Geometry check sheet. Reference: the model listing, model coordinates, mm. Face numbers are marked on the shaded views. Coordinates: 2 decimals unless noted, no trailing zeros. Write each loop counter-clockwise with the first axis right and the second up, starting at its lowest first coordinate (ties: lowest second). Pieces come first, ordered by that corner, then holes.
from build123d import *

# Parameters (mm, degrees)
SKETCH1_R           = 14
SKETCH1_R_2         = 5
BOSS_EXTRUDE1_DEPTH = 38
SKETCH2_R           = 8
SKETCH2_R_2         = 3
BOSS_EXTRUDE2_DEPTH = 16
SKETCH3_R           = 2.5
CUT_EXTRUDE1_DEPTH  = 21
SKETCH4_R           = 2.15
SKETCH4_R_2         = 2.5
CUT_EXTRUDE2_DEPTH  = 21
CUT_EXTRUDE3_DEPTH  = 1
FILLET2_R           = 0.2


with BuildPart() as part:
    # Sketch1 → Boss-Extrude1 (new body)
    with BuildSketch(Plane(origin=(0, 0, 0), x_dir=(1, 0, 0), z_dir=(0, 1, 0))):
        with BuildLine():
            Line((40, 57), (-40, 57))
            ThreePointArc((-40, 57), (-58.987886037, 46.111263827), (-59.17994648, 24.223653075))
            Line((-59.17994648, 24.223653075), (-47.255332989, 3))
            Line((-47.255332989, 3), (-32.311027529, 3))
            ThreePointArc((-32.311027529, 3), (32.415238263, -1.501608583), (-32.45, 0))
            Line((-32.45, 0), (-47.255332989, 0))
            Line((-47.255332989, 0), (-47.255332989, -10))
            Line((-47.255332989, -10), (-41.255332989, -10))
            ThreePointArc((-41.255332989, -10), (-4.643586709, -42.195255687), (38.093342034, -18.732319468))
            Line((38.093342034, -18.732319468), (59.742132503, 25.291848568))
            ThreePointArc((59.742132503, 25.291848568), (58.675911377, 46.627997861), (40, 57))
        make_face()
        with Locations((-40, 35)):
            Circle(SKETCH1_R, mode=Mode.SUBTRACT)
        with Locations((0, 44)):
            Circle(SKETCH1_R_2, mode=Mode.SUBTRACT)
        with Locations((40, 35)):
            Circle(SKETCH1_R, mode=Mode.SUBTRACT)
    extrude(amount=BOSS_EXTRUDE1_DEPTH)


with BuildPart() as body_2:
    # Sketch2 → Boss-Extrude2 (new body)
    with BuildSketch(Plane(origin=(0, 38, 0), x_dir=(1, 0, 0), z_dir=(0, 1, 0))):
        with BuildLine():
            Line((-40, 27), (40, 27))
            ThreePointArc((40, 27), (45.282843577, 28.992374534), (47.934336402, 33.977109066))
            Line((47.934336402, 33.977109066), (50, 50))
            Line((50, 50), (50, 58))
            Line((50, 58), (-50, 58))
            Line((-50, 58), (-50, 50))
            Line((-50, 50), (-47.934336402, 33.977109066))
            ThreePointArc((-47.934336402, 33.977109066), (-45.282843577, 28.992374534), (-40, 27))
        make_face()
        with Locations((0, 44)):
            Circle(SKETCH2_R, mode=Mode.SUBTRACT)
        with Locations((-40, 35)):
            Circle(SKETCH2_R_2, mode=Mode.SUBTRACT)
        with Locations((40, 35)):
            Circle(SKETCH2_R_2, mode=Mode.SUBTRACT)
    extrude(amount=BOSS_EXTRUDE2_DEPTH)

    # Sketch3 → Cut-Extrude1 (cut)
    with BuildSketch(Plane(origin=(0, 0, -58), x_dir=(-1, 0, 0), z_dir=(0, 0, -1))):
        with Locations((-40, 46)):
            Circle(SKETCH3_R)
        with Locations((40, 46)):
            Circle(SKETCH3_R)
    extrude(amount=-CUT_EXTRUDE1_DEPTH, mode=Mode.SUBTRACT)

    # Sketch4 → Cut-Extrude2 (cut)
    with BuildSketch(Plane.XZ.offset(-38)):
        with Locations((-21, -33.5)):
            Circle(SKETCH4_R)
        with Locations((-21, -51.5)):
            Circle(SKETCH4_R)
        with Locations((21, -51.5)):
            Circle(SKETCH4_R_2)
        with Locations((21, -33.5)):
            Circle(SKETCH4_R_2)
    extrude(amount=-CUT_EXTRUDE2_DEPTH, mode=Mode.SUBTRACT)

    # Sketch6 → Cut-Extrude3 (cut)
    with BuildSketch(Plane.XY.offset(-27)):
        Polygon((-6.118033989, 44), (-6.118033989, 50), (-9.618033989, 50), (-9.618033989, 42), (-3.618033989, 42), (0.381966011, 50), (-3.118033989, 50), align=None)
        Polygon((9.618033989, 50), (2.618033989, 50), (1.518033989, 47.8), (5.018033989, 47.8), (2.718033989, 43.2), (0.118033989, 42), (2.118033989, 42), (5.618033989, 42), (7.618033989, 42), (6.218033989, 43.2), align=None)
    extrude(amount=-CUT_EXTRUDE3_DEPTH, mode=Mode.SUBTRACT)

    # Fillet2
    fillet2_edges = [body_2.edges().sort_by_distance(p)[0] for p in [
        (7.618033989, 42, -27.5),
        (0.118033989, 42, -27.5),
        (2.718033989, 43.2, -27.5),
        (5.018033989, 47.8, -27.5),
        (1.518033989, 47.8, -27.5),
        (2.618033989, 50, -27.5),
        (9.618033989, 50, -27.5),
        (6.218033989, 43.2, -27.5),
        (-6.118033989, 50, -27.5),
        (-6.118033989, 44, -27.5),
        (-3.118033989, 50, -27.5),
        (0.381966011, 50, -27.5),
        (-3.618033989, 42, -27.5),
        (-9.618033989, 42, -27.5),
        (-9.618033989, 50, -27.5),
    ]]
    fillet(fillet2_edges, radius=FILLET2_R)


solid = body_2.part
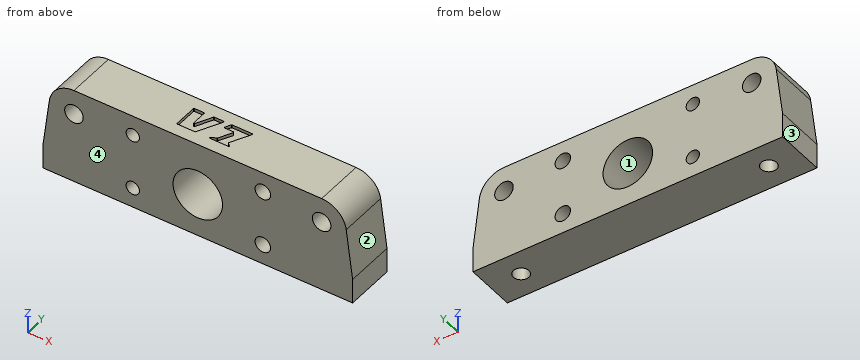
1. Draft check along X on the marked faces 1, 2, 3 and 4. Enter one of: released by +X, released by -X, zero draft, split by the parting line, or undercut.
Computed values:
face 1: undercut
face 2: released by +X
face 3: released by -X
face 4: zero draft
2. Sectioned sample at B-B, the plane y = 39.5. Record the boundary of the cut face in (x, z), and give its area (3 significant figures).
Computed values:
outline: (-50, -58) - (50, -58) - (50, -50) - (47.93, -33.98) arc R8 ccw to (40, -27) - (-40, -27) arc R8 ccw to (-47.93, -33.98) - (-50, -50) - close; hole circle Ø6 at (-40, -35); hole circle Ø4.3 at (-21, -51.5); hole circle Ø4.3 at (-21, -33.5); hole circle Ø16 at (0, -44); hole circle Ø5 at (21, -51.5); hole circle Ø5 at (21, -33.5); hole circle Ø6 at (40, -35)
area: 2,690 mm2
3. Sectioned sample at D-D, the plane x = -1.5. Record the boundary of the cut face in (y, z).
Computed values:
outline: (38, -58) - (54, -58) - (54, -51.86) - (38, -51.86) - close; (38, -36.14) - (54, -36.14) - (54, -27) - (50, -27) - (50, -28) - (46.24, -28) - (46.24, -27) - (38, -27) - close
4. Sectioned sample at A-A, the plane x = -21. Record the boundary of the cut face in (y, z), and give its area (3 significant figures).
Computed values:
outline: (38, -58) - (54, -58) - (54, -53.65) - (38, -53.65) - close; (38, -49.35) - (54, -49.35) - (54, -35.65) - (38, -35.65) - close; (38, -31.35) - (54, -31.35) - (54, -27) - (38, -27) - close
area: 358 mm2
5. Sectioned sample at C-C, the plane z = -39. Record the boundary of the cut face in (x, y) (3 decimals), and give its area (3 significant figures).
Computed values:
outline: (-48.582, 38) - (-6.245, 38) - (-6.245, 54) - (-48.582, 54) - close; (6.245, 38) - (48.582, 38) - (48.582, 54) - (6.245, 54) - close; hole circle Ø5 at (-40, 46); hole circle Ø5 at (40, 46)
area: 1,320 mm2
6. Gauge pin test, flat ends, axial feed: pin 1 Ø1 at (y, z) = (48.5, -41.5) entering from -X; pin 2 Ø5 at (y, z) = (45, -45) entering from -X; pin 3 Ø9.5 at (x, z) = (40, -35) entering from -Y. Record the tip position at first contact, or that the pin passes through.
Computed values:
pin 1: stops at x = -48.97
pin 2: stops at x = -49.68
pin 3: stops at y = 38
7. Thickness scan on line 1 along Z through (x, y) = (-21, 49.75); line 2 along Z through (x, y) = (21, 49.5); line 3 along Z through (x, y) = (-40, 49.5). Record the ranges inside material, lowest first.
Computed values:
line 1: z = -58 to -53.65, -49.35 to -35.65, -31.35 to -27
line 2: z = -58 to -54, -49 to -36, -31 to -27
line 3: z = -58 to -38, -32 to -27
